Design review of the part built by this model. Coordinates are the model's own, in mm. Face numbers are marked on the shaded views. Round coordinates to 2 decimals unless told otherwise and drop trailing zeros. Order: outer loops, then holes, each group sorted by start corner. A loop starts at its lowest first (then second) coordinate and runs counter-clockwise, first axis right, second up. Notation, with made-up numbers: (54.25, 59) - (67.25, 59) arc R18 ccw to (67.25, 80) - close; hole circle Ø11 at (85, -28). An arc over 180 degrees is marked (long way). Use CSV: the item, a comma, the result in double quotes. Start each with the question number.
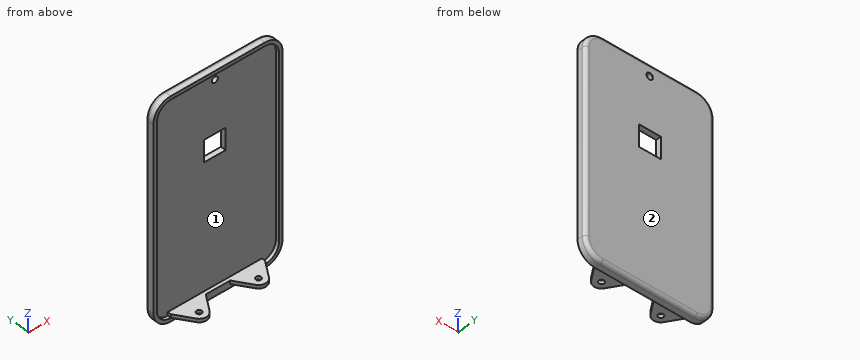
Autodesk Inventor part; units mm, degrees
ref_plane "YZ Plane" through (0, 0, 0) normal (1, 0, 0) x (0, 1, 0)
ref_plane "XZ Plane" through (0, 0, 0) normal (0, 1, 0) x (-1, 0, 0)
ref_plane "XY Plane" through (0, 0, 0) normal (0, 0, 1) x (1, 0, 0)
sketch "Sketch1" plane through (0, 0, 0) normal (0, 1, 0) x (-1, 0, 0)
  line L0 (10, 0) -> (64, 0)
  line L1 (74, -10) -> (74, -115)
  line L2 (64, -125) -> (10, -125)
  line L3 (0, -115) -> (0, -10)
  arc A0 (74, -10) -> (64, 0) centre (64, -10) ccw
  arc A1 (10, 0) -> (0, -10) centre (10, -10) ccw
  arc A2 (0, -115) -> (10, -125) centre (10, -115) ccw
  arc A3 (64, -125) -> (74, -115) centre (64, -115) ccw
  point P0 (0, 0)
  point P1 (74, -125)
  point P2 (0, -125)
  dimension "d0" = 125
  dimension "d1" = 74
  dimension "d2" = 10
extrude "Extrusion1" add sketch "Sketch1" along normal blind 3
sketch "Sketch3" plane through (0, 0, 0) normal (0, -1, 0) x (1, 0, 0)
  line L0 (-64, 0) -> (-10, 0)
  arc A0 (-64, 0) -> (-74, -10) centre (-64, -10) ccw
  line L1 (-74, -115) -> (-74, -10)
  arc A1 (-74, -115) -> (-64, -125) centre (-64, -115) ccw
  line L2 (-10, -125) -> (-64, -125)
  arc A2 (-10, -125) -> (0, -115) centre (-10, -115) ccw
  line L3 (0, -10) -> (0, -115)
  arc A3 (0, -10) -> (-10, 0) centre (-10, -10) ccw
  line L4 (-10, -2) -> (-64, -2)
  line L5 (-2, -10) -> (-2, -115)
  line L6 (-6.1409, -124.2254) -> (-6.1409, -125)
  line L7 (-72, -115) -> (-72, -10)
  line L8 (-10, -123) -> (-64, -123)
  arc A4 (-2, -10) -> (-10, -2) centre (-10, -10) ccw
  arc A5 (-64, -2) -> (-72, -10) centre (-64, -10) ccw
  arc A6 (-72, -115) -> (-64, -123) centre (-64, -115) ccw
  arc A7 (-10, -123) -> (-2, -115) centre (-10, -115) ccw
  point P0 (0, 0)
  dimension "d5" = 2
  dimension "d6" = 2
  dimension "d7" = 2
  dimension "d8" = 2
  dimension "d10" = 8
extrude "Extrusion2" add sketch "Sketch3" along normal blind 2
sketch "Sketch6" plane through (0, 0, 0) normal (0, -1, 0) x (1, 0, 0)
  arc A0 (-2, -10) -> (-10, -2) centre (-10, -10) ccw
  line L0 (-10, -2) -> (-64, -2)
  arc A1 (-64, -2) -> (-72, -10) centre (-64, -10) ccw
  line L1 (-72, -10) -> (-72, -115)
  arc A2 (-72, -115) -> (-64, -123) centre (-64, -115) ccw
  line L2 (-64, -123) -> (-10, -123)
  arc A3 (-10, -123) -> (-2, -115) centre (-10, -115) ccw
  line L3 (-2, -115) -> (-2, -10)
  line L4 (-43.25, -49.5) -> (-30.75, -49.5)
  line L5 (-30.75, -49.5) -> (-30.75, -37)
  line L6 (-30.75, -37) -> (-43.25, -37)
  line L7 (-43.25, -37) -> (-43.25, -49.5)
  line L8 (-30.75, -43.25) -> (-2, -43.25)
  line L9 (-43.25, -43.25) -> (-72, -43.25)
  line L10 (-72, -115) -> (-72, -10)
  point P0 (0, 0)
  dimension "d28" = 12.5
  dimension "d29" = 12.5
  dimension "d41" = 35
extrude "Extrusion4" cut sketch "Sketch6" against normal up to next contours L5 L4 L7 L6
fillet "Fillet1" radius 2 8 edges at (-2.9289, 3, -122.0711) (-37, 3, -125) (-71.0711, 3, -122.0711) (-74, 3, -62.5) (-71.0711, 3, -2.9289) (-37, 3, 0) (-2.9289, 3, -2.9289) (0, 3, -62.5)
ref_plane "Work Plane1" through (-10, 0, -123) normal (0, 0, 1) x (1, 0, 0)
sketch "Sketch8" plane through (-10, 0, -123) normal (0, 0, 1) x (1, 0, 0)
  line L0 (-54, 0) -> (0, 0)
  line L1 (-54, 0) -> (-54, -2)
  line L2 (0, -2) -> (-54, -2)
  line L3 (0, 0) -> (0, -2)
  circle A0 centre (-10, -9) radius 4.5
  line L4 (0, -2) -> (-54, -2)
  line L5 (-27, -2) -> (-27, -24.2121)
  line L6 (0, 0) -> (0, -2)
  line L7 (0, -2) -> (-6.2421, -11.4755)
  line L8 (-13.7579, -11.4755) -> (-20, -2)
  circle A1 centre (-10, -9) radius 1.5
  line L9 (-54, 0) -> (-54, -2)
  circle A2 centre (-44, -9) radius 4.5
  line L10 (-54, 0) -> (-54, -2)
  line L11 (-54, -2) -> (-47.7579, -11.4755)
  line L12 (-40.2421, -11.4755) -> (-34, -2)
  circle A3 centre (-44, -9) radius 1.5
  line L13 (-34, -2) -> (-54, -2)
  point P0 (10, 0)
  dimension "d34" = 7
  dimension "d35" = 9
  dimension "d36" = 10
  dimension "d37" = 10
  dimension "d38" = 3
extrude "Extrusion5" add sketch "Sketch8" along normal blind 2
sketch "Sketch10" plane through (0, 0, 0) normal (0, -1, 0) x (1, 0, 0)
  line L0 (-10, -2) -> (-64, -2)
  line L1 (-37, -2) -> (-37, -7)
  circle A0 centre (-37, -7) radius 1.75
  point P0 (0, 0)
  dimension "d42" = 5
  dimension "d43" = 3.5
extrude "Extrusion6" cut sketch "Sketch10" against normal up to surface (3 mm away)
fillet "Fillet2" radius 0.25 1 edges at (-38.75, 3, -7)
properties part number "Cover" material "PC/ABS Plastic"
Q1. Take a section at B-B (y = -4). State the section outline as (x, z) points.
Q2. The part is to be moulded in two halves that separate along X. For the marked faces 1 and 2, say which applies: +X half, -X half, draft (parallel to the pull), parting line (faces both ways), or undercut.
Q3. For L1, parallel to Z at x = -37, y = 1.1; L2, parallel to Z at x = -37, y = 1.95; L3, parallel to Y at x = -33, z = -85, list the stretches that pass through material, from the lowest coordinate up. Write a range as [from, to].
Q4. Clearance check with flat-ended pins moving along their axes: pin 1 (0.6 mm diameter, centred on y = -0.5, z = -121.5, fed in from -X); pin 2 (2 mm diameter, centred on y = -1, z = -45, fed in from +X); pin 3 (0.6 mm diameter, centred on y = -1, z = -121.5, fed in from +X); pin 4 (1.5 mm diameter, centred on x = -8.5, z = -94, fed in from -Y). State where each tip first meets the part, or that it passes through.
Q5. Take a section at C-C (x = -37). State the section outline as (y, z) points, plus the area to 3 significant figures.
Q6. Take a section at D-D (x = -54). State the section outline as (y, z) points.
Q7. Take a section at A-A (z = -42). State the section outline as (x, y) points, plus the area to 3 significant figures.
Findings below:
1,outline,"(-62.68, -123) - (-45.32, -123) - (-45.32, -121) - (-62.68, -121) - close; (-28.68, -123) - (-11.32, -123) - (-11.32, -121) - (-28.68, -121) - close"
2,face 1,"undercut"
2,face 2,"draft"
3,L1,"z = [-125, -49.5], [-37, -8.75], [-5.25, 0]"
3,L2,"z = [-124.76, -49.5], [-37, -8.75], [-5.25, -0.24]"
3,L3,"y = [0, 3]"
4,pin 1,"stops at x = -71.85"
4,pin 2,"stops at x = 0"
4,pin 3,"stops at x = -2.15"
4,pin 4,"stops at y = 0"
5,outline,"(-2, -125) - (1, -125) arc R2 ccw to (3, -123) - (3, -49.5) - (0, -49.5) - (0, -121) - (-2, -121) - close; (-2, -2) - (0, -2) - (0, -5.25) - (2.75, -5.25) arc R0.25 ccw to (3, -5) - (3, -2) arc R2 ccw to (1, 0) - (-2, 0) - close; (0, -37) - (3, -37) - (3, -9) arc R0.25 ccw to (2.75, -8.75) - (0, -8.75) - close"
5,area,"337 mm^2"
6,outline,"(-13.5, -123) - (-10.5, -123) - (-10.5, -121) - (-13.5, -121) - close; (-7.5, -123) - (-2, -123) - (-2, -125) - (1, -125) arc R2 ccw to (3, -123) - (3, -2) arc R2 ccw to (1, 0) - (-2, 0) - (-2, -2) - (0, -2) - (0, -121) - (-7.5, -121) - close"
7,outline,"(-74, -2) - (-72, -2) - (-72, 0) - (-43.25, 0) - (-43.25, 3) - (-72, 3) arc R2 ccw to (-74, 1) - close; (-30.75, 0) - (-2, 0) - (-2, -2) - (0, -2) - (0, 1) arc R2 ccw to (-2, 3) - (-30.75, 3) - close"
7,area,"191 mm^2"
